from build123d import *

# Parameters (mm, degrees)
SKETCH1_W           = 248.25
SKETCH1_H           = 19.05
BOSS_EXTRUDE1_DEPTH = 38.1
HOLE1_D             = 3.175
HOLE1_DEPTH         = 31.75
HOLE1_CSINK_D       = 10.16
HOLE1_CSINK_ANGLE   = 82
HOLE1_TIP           = 0.953866233
HOLE2_D             = 3.175
HOLE2_DEPTH         = 57.15
HOLE2_CSINK_D       = 10.16
HOLE2_CSINK_ANGLE   = 82
HOLE2_TIP           = 0.953866233


with BuildPart() as part:
    # Sketch1 → Boss-Extrude1 (new body)
    with BuildSketch(Plane.XY):
        with Locations((124.125, 47.625)):
            Rectangle(SKETCH1_W, SKETCH1_H)
    extrude(amount=BOSS_EXTRUDE1_DEPTH)

    # Hole1
    with Locations(Plane(origin=(-1090.512770337, -52.974999997, -12.7), x_dir=(0, 1, 0), z_dir=(0, 0, -1))):
        with Locations((-100.332047386, 1313.362770337), (100.599999997, 1313.362770337), (100.599999997, 1115.912770337), (100.599999997, 1214.637770337), (-100.332047386, 1214.637770337), (-100.332047386, 1115.912770337)):
            CounterSinkHole(HOLE1_D / 2, HOLE1_CSINK_D / 2, depth=HOLE1_DEPTH, counter_sink_angle=HOLE1_CSINK_ANGLE)
            with Locations((0, 0, -(HOLE1_DEPTH + HOLE1_TIP / 2))):  # 118° drill point
                Cone(0, HOLE1_D / 2, HOLE1_TIP, mode=Mode.SUBTRACT)

    # Hole2
    with Locations(Plane(origin=(-1090.512770337, 57.15, -415.792401694), x_dir=(0.374606593, 0, 0.927183855), z_dir=(0, 1, 0))):
        with Locations((848.944412528, 940.413642522), (885.927448463, 1031.949868564), (867.435930496, 986.181755543), (830.452894561, 894.645529501)):
            CounterSinkHole(HOLE2_D / 2, HOLE2_CSINK_D / 2, depth=HOLE2_DEPTH, counter_sink_angle=HOLE2_CSINK_ANGLE)
            with Locations((0, 0, -(HOLE2_DEPTH + HOLE2_TIP / 2))):  # 118° drill point
                Cone(0, HOLE2_D / 2, HOLE2_TIP, mode=Mode.SUBTRACT)


solid = part.part
Geometry check sheet. Reference: the model listing, model coordinates, mm. Round coordinates to 2 decimals unless told otherwise and drop trailing zeros. Use one line per item in the form item = value.
1. Scan lines: line 1 along X through (y, z) = (46, 19.05); line 2 along X through (y, z) = (48.5, 9); line 3 along X through (y, z) = (55.25, 17). Record each from-to range of solid material in increasing order. Write a range as from..to.
Working result:
line_1 = 0..48.49, 51.67..97.86, 101.03..147.22, 150.39..196.58, 199.76..248.25
line_2 = 0..24.08, 26.72..122.8, 125.45..221.53, 224.17..248.25
line_3 = 0..47.33, 52.83..96.7, 102.19..146.06, 151.55..195.42, 200.92..248.25
2. Mould release check, pull along Z, two halves, no side actions. Record for faces 1 (the face through (150.51, 53.33, 18.61)), 2 (the face through (122, 48, 38.1)), 3 (the face through (0, 47, 19)): pulls with the +Z half, pulls with the -Z half, needs draft (parallel to the pull), parting line crosses it, or undercut.
Working result:
face_1 = undercut
face_2 = pulls with the +Z half
face_3 = needs draft
3. Go/stop test with flat-tipped pins: pin 1 (1.9 mm diameter, centred on x = 99.44, z = 19.05, fed in from -Y); pin 2 (1.9 mm diameter, centred on x = 25.4, y = 47.625, fed in from -Z). Record where each tip stops, or that it passes through.
Working result:
pin_1 = through
pin_2 = 19.43
